```python
from build123d import *

# Parameters (mm, degrees)
F0_R      = 3
F0_W      = 20
F0_H      = 2
F1_DEPTH  = 2
F0_R_2    = 0.5
F2_DEPTH  = 13
F3_DEPTH  = 23
F4_DEPTH  = 6
F5_R      = 1.5
F6_DEPTH  = 25
F7_R      = 1.5
F8_DEPTH  = 5
F9_R      = 1.5
F10_DEPTH = 5


with BuildPart() as f1:
    # F0 (on Top) → F1 (new body)
    with BuildSketch(Plane.XY):
        with BuildLine():
            Line((-20.860016, 43.776053), (-140.860016, 43.776053))
            Line((-140.860016, 43.776053), (-140.860016, 38.776053))
            Line((-140.860016, 38.776053), (-170.860016, 38.776053))
            Line((-170.860016, 38.776053), (-170.860016, -61.223947))
            Line((-170.860016, -61.223947), (-140.860016, -61.223947))
            Line((-140.860016, -61.223947), (-140.860016, -66.223947))
            Line((-140.860016, -66.223947), (-20.860016, -66.223947))
            Line((-20.860016, -66.223947), (-20.860016, -56.223947))
            Line((-20.860016, -56.223947), (9.139984, -56.223947))
            ThreePointArc((9.139984, -56.223947), (11.639984, -53.723947), (14.139984, -56.223947))
            Line((14.139984, -56.223947), (19.139984, -56.223947))
            Line((19.139984, -56.223947), (19.139984, 33.776053))
            Line((19.139984, 33.776053), (14.139984, 33.776053))
            ThreePointArc((14.139984, 33.776053), (11.639984, 31.276053), (9.139984, 33.776053))
            Line((9.139984, 33.776053), (-20.860016, 33.776053))
            Line((-20.860016, 33.776053), (-20.860016, 43.776053))
        make_face()
        with Locations((-157.860016, -56.223947)):
            Circle(F0_R, mode=Mode.SUBTRACT)
        with Locations((-103.860016, -62.223947)):
            Circle(F0_R, mode=Mode.SUBTRACT)
        with Locations((-103.860016, -45.723947)):
            Circle(F0_R, mode=Mode.SUBTRACT)
        with Locations((-115.650242, -35.223947)):
            Rectangle(F0_W, F0_H, mode=Mode.SUBTRACT)
        Polygon((-157.64454, -24.237227), (-157.64454, 25.332287), (-75.020161, 25.332287), (-75.020161, 18.624624), (1.898053, 18.624624), (1.898053, -5.519149), (-18.613469, -5.519149), (-18.613469, -30.519149), (-48.526108, -30.519149), (-48.526108, -5.519149), (-75.020161, -5.519149), (-75.020161, -24.237227), (-75.020161, -54.237227), (-99.020161, -54.237227), (-99.020161, -24.237227), (-136.492044, -24.237227), (-136.492044, -40.902838), (-157.64454, -40.902838), align=None, mode=Mode.SUBTRACT)
        with Locations((-66.860016, -62.223947)):
            Circle(F0_R, mode=Mode.SUBTRACT)
        with Locations((-66.860016, -45.723947)):
            Circle(F0_R, mode=Mode.SUBTRACT)
        with Locations((-37.650242, -35.641791)):
            Rectangle(F0_W, F0_H, mode=Mode.SUBTRACT)
        with Locations((-60.860016, -20.223947)):
            Circle(F0_R, mode=Mode.SUBTRACT)
        with Locations((-2.860016, -20.223947)):
            Circle(F0_R, mode=Mode.SUBTRACT)
        with Locations((-157.860016, 33.776053)):
            Circle(F0_R, mode=Mode.SUBTRACT)
        with Locations((-115.860016, 36.776053)):
            Rectangle(F0_W, F0_H, mode=Mode.SUBTRACT)
        with Locations((-60.860016, 28.776053)):
            Circle(F0_R, mode=Mode.SUBTRACT)
        with Locations((-2.860016, 28.776053)):
            Circle(F0_R, mode=Mode.SUBTRACT)
    extrude(amount=F1_DEPTH)

    # F0 (on Top) → F2 (join)
    with BuildSketch(Plane.XY):
        with Locations((-157.860016, 33.776053)):
            Circle(F0_R)
        with Locations((-157.860016, 33.776053)):
            Circle(F0_R_2, mode=Mode.SUBTRACT)
        with Locations((-157.860016, -56.223947)):
            Circle(F0_R)
        with Locations((-157.860016, -56.223947)):
            Circle(F0_R_2, mode=Mode.SUBTRACT)
    extrude(amount=F2_DEPTH)

    # F0 (on Top) → F3 (join)
    with BuildSketch(Plane.XY):
        with Locations((-115.650242, -35.223947)):
            Rectangle(F0_W, F0_H)
        with Locations((-115.860016, 36.776053)):
            Rectangle(F0_W, F0_H)
        with Locations((-37.650242, -35.641791)):
            Rectangle(F0_W, F0_H)
    extrude(amount=F3_DEPTH)

    # F0 (on Top) → F4 (join)
    with BuildSketch(Plane.XY):
        with Locations((-60.860016, 28.776053)):
            Circle(F0_R)
        with Locations((-60.860016, 28.776053)):
            Circle(F0_R_2, mode=Mode.SUBTRACT)
        with Locations((-2.860016, 28.776053)):
            Circle(F0_R)
        with Locations((-2.860016, 28.776053)):
            Circle(F0_R_2, mode=Mode.SUBTRACT)
        with Locations((-2.860016, -20.223947)):
            Circle(F0_R)
        with Locations((-2.860016, -20.223947)):
            Circle(F0_R_2, mode=Mode.SUBTRACT)
        with Locations((-60.860016, -20.223947)):
            Circle(F0_R)
        with Locations((-60.860016, -20.223947)):
            Circle(F0_R_2, mode=Mode.SUBTRACT)
        with Locations((-66.860016, -45.723947)):
            Circle(F0_R)
        with Locations((-66.860016, -45.723947)):
            Circle(F0_R_2, mode=Mode.SUBTRACT)
        with Locations((-66.860016, -62.223947)):
            Circle(F0_R)
        with Locations((-66.860016, -62.223947)):
            Circle(F0_R_2, mode=Mode.SUBTRACT)
        with Locations((-103.860016, -62.223947)):
            Circle(F0_R)
        with Locations((-103.860016, -62.223947)):
            Circle(F0_R_2, mode=Mode.SUBTRACT)
        with Locations((-103.860016, -45.723947)):
            Circle(F0_R)
        with Locations((-103.860016, -45.723947)):
            Circle(F0_R_2, mode=Mode.SUBTRACT)
    extrude(amount=F4_DEPTH)

    # F5 (on face) → F6 (cut)
    with BuildSketch(Plane.XZ.offset(36.223947)):
        with Locations((-115.650242, 20.5)):
            Circle(F5_R)
    extrude(amount=-F6_DEPTH, mode=Mode.SUBTRACT)

    # F7 (on face) → F8 (cut)
    with BuildSketch(Plane(origin=(0, 37.776053, 0), x_dir=(-1, 0, 0), z_dir=(0, 1, 0))):
        with Locations((115.860016, 20.5)):
            Circle(F7_R)
    extrude(amount=-F8_DEPTH, mode=Mode.SUBTRACT)

    # F9 (on face) → F10 (cut)
    with BuildSketch(Plane.XZ.offset(36.641791)):
        with Locations((-37.650242, 20.5)):
            Circle(F9_R)
    extrude(amount=-F10_DEPTH, mode=Mode.SUBTRACT)


solid = f1.part
```
Here's how the part is built. I have some questions about the finished solid (model axes, mm). A direction names the side the tool comes from. Round coordinates to 2 decimals unless told otherwise and drop trailing zeros. Loops run counter-clockwise (first coordinate to the right, second up) from the corner with the lowest first, then second, coordinate; pieces in that order, holes last.
1. Will these pins go through, and if not, where does the flat tip stop? pin 1 (2 mm diameter, centred on y = 36.5, z = 17.5, fed in from +X); pin 2 (4 mm diameter, centred on x = -119.5, z = 14, fed in from +Y); pin 3 (3 mm diameter, centred on x = -104.5, y = -47, fed in from +Z).
Answers:
pin 1: stops at x = -105.86
pin 2: stops at y = 37.78
pin 3: stops at z = 6
2. Suppose I cut it at B-B, the plane x = -24.5. Please give me the cut outline in (y, z).
Answers:
outline: (-66.22, 0) - (-30.52, 0) - (-30.52, 2) - (-66.22, 2) - close; (18.62, 0) - (43.78, 0) - (43.78, 2) - (18.62, 2) - close
3. Suppose I cut it at A-A, the plane y = -3. Please give me the cut outline in (x, z).
Answers:
outline: (-170.86, 0) - (-157.64, 0) - (-157.64, 2) - (-170.86, 2) - close; (1.9, 0) - (19.14, 0) - (19.14, 2) - (1.9, 2) - close
4. Suppose I cut it at C-C, the plane z = 15.5. Please give me the cut outline in (x, y).
Answers:
outline: (-125.86, 35.78) - (-105.86, 35.78) - (-105.86, 37.78) - (-125.86, 37.78) - close; (-125.65, -36.22) - (-105.65, -36.22) - (-105.65, -34.22) - (-125.65, -34.22) - close; (-47.65, -36.64) - (-27.65, -36.64) - (-27.65, -34.64) - (-47.65, -34.64) - close
5. Thinking about a two-plate mould opening in X: for faces 1 (the face through (-67, -63, 6)), 2 (the face through (-58, 29.68, 3.97)), 3 (the face through (-101, -61.32, 3.97)), which applies, released by +X, released by -X, zero draft, split by the parting line, or undercut?
Answers:
face 1: zero draft
face 2: undercut
face 3: undercut
6. For faces 4 (the face through (-38, -34.642, 12)), 5 (the face through (-64, -44.82, 3.97)), 6 (the face through (-38, -36.642, 12)), 7 (the face through (-61, 28, 6)), which set-ups out of +Z, -Z, +X, -X, +Y, -Y let a thin tool reach every point of the face, with its end or its side?
Answers:
face 4: +Z, +X, +Y
face 5: +Z
face 6: +Z, +X, -X, -Y
face 7: +Z, +X, +Y, -Y
7. If I drill on probe 1 along X at (y, z) = (-33.5, 1.75); probe 2 along Y at (x, z) = (-114, 17.75); probe 3 along Y at (x, z) = (-106.5, 3.5), over which ranges is the centre line in solid material (lowest first)?
Answers:
probe 1: x = -170.86 to -157.64, -136.49 to -99.02, -75.02 to 19.14
probe 2: y = -36.22 to -34.22, 35.78 to 37.78
probe 3: y = -63.65 to -60.8, -47.15 to -44.3, -36.22 to -34.22, 35.78 to 37.78
